```python
from build123d import *

# Parameters (mm, degrees)
F0_R          = 16
F0_R_2        = 14
F1_DEPTH      = 32
F2_R          = 14
F3_DEPTH      = 30
F4_R          = 1
F5_W          = 6
F5_H          = 6
F6_DEPTH      = 35.5
F6_DEPTH_BACK = 16.5


# Not quite as in the source:
# - a feature names something its author has since deleted; it is built from what else it names


with BuildPart() as f1:
    # F0 (on Front) → F1 (new body)
    with BuildSketch(Plane.XZ):
        with Locations((-13.5661968961, 9.2302449048)):
            Circle(F0_R)
        with Locations((-13.5661968961, 9.2302449048)):
            Circle(F0_R_2, mode=Mode.SUBTRACT)
        with Locations((-13.5661968961, 9.2302449048)):
            Circle(F0_R_2)
    extrude(amount=F1_DEPTH)

    # F2 (on face) → F3 (cut)
    with BuildSketch(Plane(origin=(0, 0, 0), x_dir=(-1, 0, 0), z_dir=(0, 1, 0))):
        with Locations((13.5661968961, 9.2302449048)):
            Circle(F2_R)
    extrude(amount=-F3_DEPTH, mode=Mode.SUBTRACT)

    # F4
    f4_edges = [f1.edges().sort_by_distance(p)[0] for p in [
        (-29.566197, -32, 9.230245),
    ]]
    fillet(f4_edges, radius=F4_R)

    # F5 (on Right) → F6 (cut, two sides)
    with BuildSketch(Plane.YZ) as f6_sk:
        with Locations((-7, 8.7253677193)):
            Rectangle(F5_W, F5_H)
    extrude(amount=-F6_DEPTH, mode=Mode.SUBTRACT)
    extrude(f6_sk.sketch, amount=F6_DEPTH_BACK, mode=Mode.SUBTRACT)


solid = f1.part
```
CAD build for the part. Positions are in the model's coordinates, mm. A direction names the side the tool comes from. Give positions to 0.01 mm unless a question says otherwise; leave off trailing zeros. Loops run counter-clockwise (first coordinate to the right, second up) from the corner with the lowest first, then second, coordinate; pieces in that order, holes last. Notation, with made-up numbers: M -7.5,42 L 15.5,42 A32 ccw 15.5,78 Z; hole C 73,62.25 d11. An arc over 180 degrees is marked long. Use one line per item in the form item = value.
Item 1: Slice it at B-B (y = -3). List the corners of the cut face in (x, z).
Determined:
outline = C -13.57,9.23 d32; hole C -13.57,9.23 d28
Item 2: Slice it at A-A (y = -7). List the corners of the cut face in (x, z).
Determined:
outline = M -29.37,11.73 L -27.34,11.73 A14 cw 0.21,11.73 L 2.24,11.73 A16 ccw Z; M -29.18,5.73 A16 ccw 2.05,5.73 L -0.01,5.73 A14 cw -27.12,5.73 Z
Item 3: Which spindle directions (+Z, -Z, +X, -X, +Y, -Y) get a long thin tool onto all of the face, cutting with end or side? Do faces 1 (the face through (-26.92, -14.79, 13.44)), 2 (the face through (-14, -32, 9)), 3 (the face through (-29, -4, 9)). Say none if no direction does.
Determined:
face_1 = +Y
face_2 = +Z, -Z, +X, -X, -Y
face_3 = +X, -X
Item 4: Drill centre lines: probe 1 along Z at (x, y) = (-14, -10.5); probe 2 along Y at (x, z) = (-12.5, 3.5); probe 3 along X at (y, z) = (-20, 16.5). Where is each one in solid material? Low to high. Write a range as from..to.
Determined:
probe_1 = -6.76..-4.76, 23.22..25.22
probe_2 = -32..-30
probe_3 = -27.82..-25.53, -1.6..0.69
Item 5: Flat gauge pins, fed straight in: pin 1 (1.6 mm diameter, centred on x = 1.5, y = -8.5, fed in from -Z); pin 2 (12 mm diameter, centred on x = -15, z = 4, fed in from +Y); pin 3 (4 mm diameter, centred on y = -14, z = 19, fed in from +X). Where does each tip first touch, or does it go through?
Determined:
pin_1 = 1.99
pin_2 = -30
pin_3 = 0.42
Item 6: Two-plate mould, pull along Z, no slides. Class faces 4 (the face through (-14, 0, -5)), 5 (the face through (1.695, -15.283, 14.036)), 6 (the face through (-13, -30, 9)): pulls with the +Z half, pulls with the -Z half, needs draft (parallel to the pull), parting line crosses it, or undercut.
Determined:
face_4 = needs draft
face_5 = parting line crosses it
face_6 = undercut
